Input: part model. Units: mm. Frame: model coordinates. A direction names the side the tool comes from. Round coordinates to 2 decimals unless told otherwise and drop trailing zeros. Loops run counter-clockwise (first coordinate to the right, second up) from the corner with the lowest first, then second, coordinate; pieces in that order, holes last.
1) First-contact query: pin 1 (1.5 mm diameter, centred on y = 1.5, z = -3, fed in from -X); pin 2 (0.9 mm diameter, centred on y = 2, z = -6, fed in from +X); pin 3 (1.5 mm diameter, centred on x = 18.5, z = -1, fed in from -Y); pin 4 (0.9 mm diameter, centred on y = 2, z = -37, fed in from +X). Flat tips, straight axial feed; report the tip coordinate or a pass-through.
2) Draft query along X for faces 5 (the face through (7, 2, -7)), 6 (the face through (12, 2, -55)), 7 (the face through (83.845, 1, 4)). Return one class per face: pulls with the +X half, pulls with the -X half, needs draft (parallel to the pull), parting line crosses it, or undercut.
3) Access query for faces 1 (the face through (77, 2, -37)), 2 (the face through (0, 1, -4)), 3 (the face through (70.25, 2, -26)), 4 (the face through (7, 2, -54)). Directions: +Z, -Z, +X, -X, +Y, -Y. A direction counts if a zero-diameter tool reaches every point of the face in a straight line with its end or side. Return the directions, or none.
4) Section B-B, the plane z = -5. Return loops of the section in (x, y).
5) Ray query, line 1 along Z through (x, y) = (74.5, 2.1); line 2 along X through (y, z) = (1.3, -5); line 3 along Z through (x, y) = (63, 0.9). Return the intervals inside material, ascending.
6) Section A-A, the plane x = 63. Return loops of the section in (y, z), and give its area (3 significant figures).
7) Section D-D, the plane y = 1.8. State how many separate pieces and enclosed holes the cut face has, and give its area (3 significant figures).
8) Section C-C, the plane z = 4.45. Return loops of the section in (x, y).
Autodesk Inventor part; units mm, degrees
ref_plane "YZ Plane" through (0, 0, 0) normal (1, 0, 0) x (0, 1, 0)
ref_plane "XZ Plane" through (0, 0, 0) normal (0, 1, 0) x (-1, 0, 0)
ref_plane "XY Plane" through (0, 0, 0) normal (0, 0, 1) x (1, 0, 0)
sketch "Esboço1" plane through (0, 0, 0) normal (0, 1, 0) x (-1, 0, 0)
  line L0 (0, 0) -> (-74, 0)
  line L1 (-74, 0) -> (-74, -52)
  line L2 (-74, -52) -> (0, -52)
  line L3 (0, -52) -> (0, 0)
  line L4 (-6.0465, -39.0348) -> (-22.7965, -39.0348)
  line L5 (-22.7965, -39.0348) -> (-22.7965, -36.6698)
  line L6 (-22.7965, -36.6698) -> (-6.0465, -36.6698)
  line L7 (-6.0465, -36.6698) -> (-6.0465, -39.0348)
  dimension "d0" = 74
  dimension "d1" = 52
  dimension "d22" = 16.75
  dimension "d23" = 2.365
extrude "Extrusão1" add sketch "Esboço1" along normal blind 3 contours L3 L2 L1 L0 | L4 L5 L6 L7
sketch "Esboço2" plane through (0, 3, 0) normal (0, 1, 0) x (1, 0, 0)
  line L0 (0, 52) -> (0, 0)
  line L1 (74, 52) -> (0, 52)
  line L2 (7, 52) -> (17, 52)
  line L3 (17, 52) -> (17, 55)
  line L4 (17, 55) -> (7, 55)
  line L5 (7, 55) -> (7, 52)
  line L6 (32, 52) -> (42, 52)
  line L7 (42, 52) -> (42, 55)
  line L8 (42, 55) -> (32, 55)
  line L9 (32, 55) -> (32, 52)
  line L10 (57, 52) -> (67, 52)
  line L11 (67, 52) -> (67, 55)
  line L12 (67, 55) -> (57, 55)
  line L13 (57, 55) -> (57, 52)
  line L14 (74, 0) -> (74, 52)
  point P0 (17, 52)
  point P1 (67, 52)
  point P2 (42, 52)
  point P3 (7, 53.5)
  point P4 (67, 53.5)
  point P5 (57, 53.5)
  point P6 (42, 53.5)
  point P7 (17, 53.5)
  point P8 (32, 53.5)
  point P9 (0, 26)
  dimension "d13" = 3
  dimension "d38" = 7
  dimension "d39" = 7
  dimension "d40" = 15
  dimension "d42" = 10
  dimension "d44" = 10
  dimension "d45" = 10
extrude "Extrusão2" add sketch "Esboço2" against normal blind 3
sketch "Esboço5" plane through (0, 3, 0) normal (0, 1, 0) x (1, 0, 0)
  circle A0 centre (63, 5) radius 3.1
  line L0 (0, 52) -> (0, 0)
  line L1 (7, 52) -> (0, 52)
  line L2 (74, 0) -> (74, 52)
  line L3 (0, 0) -> (74, 0)
  point P0 (3.5, 52)
  dimension "d46" = 6.2
  dimension "d113" = 11
  dimension "d114" = 52
  dimension "d116" = 5
extrude "Extrusão4" cut sketch "Esboço5" against normal blind 10
sketch "Esboço6" plane through (0, 3, 0) normal (0, 1, 0) x (1, 0, 0)
  line L0 (70.25, 13.9187) -> (74, 13.9188)
  line L1 (74, 13.9188) -> (74, 38.0813)
  line L2 (74, 38.0813) -> (70.25, 38.0813)
  line L3 (70.25, 38.0813) -> (70.25, 13.9187)
  line L4 (74, 0) -> (74, 52)
  line L5 (74, 52) -> (67, 52)
  line L6 (0, 0) -> (74, 0)
  point P0 (72.125, 38.0813)
  dimension "d49" = 3.75
  dimension "d50" = 24.1625
  dimension "d51" = 0
  dimension "d55" = 13.9187
  dimension "d100" = 13.9187
extrude "Extrusão5" cut sketch "Esboço6" against normal blind 10
sketch "Esboço7" plane through (0, 3, 0) normal (0, 1, 0) x (1, 0, 0)
  line L0 (0, 10) -> (-3, 10)
  line L1 (-3, 10) -> (-3, 20)
  line L2 (-3, 20) -> (0, 20)
  line L3 (0, 20) -> (0, 10)
  line L4 (0, 42) -> (-3, 42)
  line L5 (-3, 42) -> (-3, 32)
  line L6 (-3, 32) -> (0, 32)
  line L7 (0, 32) -> (0, 42)
  line L8 (7, 52) -> (0, 52)
  line L9 (0, 0) -> (74, 0)
  line L10 (74, 10) -> (77, 10)
  line L11 (77, 10) -> (77, 20)
  line L12 (77, 20) -> (74, 20)
  line L13 (74, 20) -> (74, 10)
  line L14 (74, 52) -> (67, 52)
  line L15 (74, 38.0813) -> (74, 52)
  line L16 (74, 42) -> (77, 42)
  line L17 (77, 42) -> (77, 32)
  line L18 (77, 32) -> (74, 32)
  line L19 (74, 32) -> (74, 42)
  line L20 (0, 0) -> (74, 0)
  point P0 (-1.5, 42)
  point P1 (7, 0)
  point P2 (-1.5, 10)
  point P3 (75.5, 42)
  point P4 (67, 0)
  point P5 (37, 0)
  point P6 (75.5, 10)
  dimension "d66" = 3
  dimension "d67" = 10
  dimension "d68" = 3
  dimension "d69" = 10
  dimension "d70" = 10
  dimension "d71" = 10
  dimension "d74" = 3
  dimension "d76" = 3
  dimension "d77" = 10
  dimension "d78" = 10
  dimension "d81" = 10
extrude "Extrusão6" add sketch "Esboço7" against normal blind 3
sketch "Esboço8" plane through (0, 0, 0) normal (0, -1, 0) x (1, 0, 0)
  line L0 (0, 0) -> (74, 0)
  line L1 (69, 0) -> (83.8454, 0)
  line L2 (83.8454, 0) -> (83.8454, 8.6)
  line L3 (74, 0) -> (74, -10)
  circle A0 centre (79.548, 4.45) radius 2.2
  line L4 (74, 0) -> (74, 8.6)
  arc A1 (74, 8.6) -> (69, 0) centre (77.4588, 0.8356) ccw
  line L5 (74, 8.6) -> (83.8454, 8.6)
  point P0 (83.8454, 4.3)
  point P1 (74, 4.3)
  dimension "d84" = 8.6
  dimension "d86" = 4.4
  dimension "d94" = 8.5
  dimension "d99" = 5
  dimension "d101" = 4.15
  dimension "d104" = 5.55
  dimension "d106" = 4.3
extrude "Extrusão7" add sketch "Esboço8" against normal blind 3
sketch "Esboço10" plane through (0, 0, 0) normal (0, -1, 0) x (1, 0, 0)
  line L0 (83.8454, 0) -> (74, 0)
  line L1 (74, 0) -> (0, 0)
  line L2 (0, 0) -> (0, 3)
  line L3 (0, 3) -> (74, 3)
  line L4 (74, 3) -> (74, 0)
  dimension "d95" = 3
extrude "Extrusão9" add sketch "Esboço10" against normal blind 3
sketch "Esboço11" plane through (0, 3, 0) normal (0, 1, 0) x (1, 0, 0)
  line L0 (13, 4) -> (7, 4)
  line L1 (7, 4) -> (7, 10)
  line L2 (7, 10) -> (13, 10)
  line L3 (13, 10) -> (13, 4)
  line L4 (0, 10) -> (0, -3)
  line L5 (0, -3) -> (69.239, -3)
  line L6 (-3, 10) -> (0, 10)
  point P0 (0, 0)
  dimension "d107" = 6
  dimension "d108" = 6
  dimension "d109" = 7
  dimension "d115" = 0
extrude "Extrusão10" cut sketch "Esboço11" against normal blind 10
properties part number "Parede_lateral_2"
Final values:
1. pin 1: stops at x = 0
1. pin 2: stops at x = 74
1. pin 3: stops at y = 0
1. pin 4: stops at x = 77
2. face 5: undercut
2. face 6: needs draft
2. face 7: pulls with the +X half
3. face 1: -Z, +X, +Y, -Y
3. face 2: +Z, -X, +Y, -Y
3. face 3: +Y, -Y
3. face 4: -Z, -X, +Y, -Y
4. outline: (0, 0) - (7, 0) - (7, 3) - (0, 3) - close; (13, 0) - (59.9, 0) - (59.9, 3) - (13, 3) - close; (66.1, 0) - (74, 0) - (74, 3) - (66.1, 3) - close
5. line 1: z = -42 to -32, -20 to -10, 0 to 8.6
5. line 2: x = 0 to 7, 13 to 59.9, 66.1 to 74
5. line 3: z = -55 to -8.1, -1.9 to 3
6. outline: (0, -55) - (3, -55) - (3, -8.1) - (0, -8.1) - close; (0, -1.9) - (3, -1.9) - (3, 3) - (0, 3) - close
6. area: 155 mm2
7. separate pieces: 1
7. enclosed holes: 3
7. area: 4,210 mm2
8. outline: (69.77, 0) - (77.35, 0) - (77.35, 3) - (69.77, 3) - close; (81.75, 0) - (83.85, 0) - (83.85, 3) - (81.75, 3) - close
